Design review of the part built by this model. Coordinates are the model's own, in mm. Give positions to 0.01 mm unless a question says otherwise; leave off trailing zeros. Answer in a Markdown table with one row per item.
```python
from build123d import *

# Parameters (mm, degrees)
ESQUISSE1_W                                    = 381
ESQUISSE1_H                                    = 381
BOSS_EXTRU_1_DEPTH                             = 3
BOSS_EXTRU_2_DEPTH                             = 3
FRAISAGE_POUR_VIS_T_TE_FRAIS_E_M31_D           = 3.4
FRAISAGE_POUR_VIS_T_TE_FRAIS_E_M31_CSINK_D     = 6.3
FRAISAGE_POUR_VIS_T_TE_FRAIS_E_M31_CSINK_ANGLE = 90


with BuildPart() as part:
    # Esquisse1 → Boss.-Extru.1 (new body)
    with BuildSketch(Plane.XY):
        with Locations((190.5, 190.5)):
            Rectangle(ESQUISSE1_W, ESQUISSE1_H)
    extrude(amount=BOSS_EXTRU_1_DEPTH)

    # Esquisse2 → Boss.-Extru.2 (add)
    with BuildSketch(Plane.XY.offset(3)):
        with BuildLine():
            Line((6.5, 3.1), (374.5, 3.1))
            ThreePointArc((374.5, 3.1), (376.904163056, 4.095836944), (377.9, 6.5))
            Line((377.9, 6.5), (377.9, 374.5))
            ThreePointArc((377.9, 374.5), (376.904163056, 376.904163056), (374.5, 377.9))
            Line((374.5, 377.9), (6.5, 377.9))
            ThreePointArc((6.5, 377.9), (4.095836944, 376.904163056), (3.1, 374.5))
            Line((3.1, 374.5), (3.1, 6.5))
            ThreePointArc((3.1, 6.5), (4.095836944, 4.095836944), (6.5, 3.1))
        make_face()
    extrude(amount=BOSS_EXTRU_2_DEPTH)

    # Fraisage pour vis à tête fraisée M31 (through all)
    with Locations(Plane(origin=(0, 0, 0), x_dir=(-1, 0, 0), z_dir=(0, 0, -1))):
        with Locations((-28.5, 5), (-82.5, 5), (-136.5, 5), (-190.5, 5), (-244.5, 5), (-298.5, 5), (-352.5, 5), (-376, 28.5), (-376, 82.5), (-376, 136.5), (-376, 190.5), (-376, 244.5), (-376, 298.5), (-376, 352.5), (-352.5, 376), (-298.5, 376), (-244.5, 376), (-190.5, 376), (-136.5, 376), (-82.5, 376), (-28.5, 376), (-5, 352.5), (-5, 298.5), (-5, 244.5), (-5, 190.5), (-5, 136.5), (-5, 82.5), (-5, 28.5)):
            CounterSinkHole(FRAISAGE_POUR_VIS_T_TE_FRAIS_E_M31_D / 2, FRAISAGE_POUR_VIS_T_TE_FRAIS_E_M31_CSINK_D / 2, counter_sink_angle=FRAISAGE_POUR_VIS_T_TE_FRAIS_E_M31_CSINK_ANGLE)


solid = part.part
```
1) The part is to be moulded in two halves that separate along Z. For faces 1 (the face through (188, 193, 0)), 2 (the face through (188, 193, 6)), say which applies: released by +Z, released by -Z, zero draft, split by the parting line, or undercut.
Geometry says:
| item | result |
|---|---|
| face 1 | released by -Z |
| face 2 | released by +Z |
2) Insertion check: P1, Ø5.5, axis at x = 298.5, y = 376, coming from the +Z side; P2, Ø4.5, axis at x = 190.5, y = 376, coming from the -Z side; P3, Ø5.5, axis at x = 376, y = 82.5, coming from the -Z side. Each pin has a flat end and moves straight along its axis. Give the tip position at first contact, or say it passes through.
Geometry says:
| item | result |
|---|---|
| P1 | z = 6 |
| P2 | z = 0.9 |
| P3 | z = 0.4 |
3) To check wall thickness, follow probe 1 along Y at (x, z) = (190.5, 4.95); probe 2 along Y at (x, z) = (190.5, 2.75). State the ranges of each line that lie inside material, in increasing order. Write a range as [from, to].
Geometry says:
| item | result |
|---|---|
| probe 1 | [3.1, 3.3], [6.7, 374.3], [377.7, 377.9] |
| probe 2 | [0, 3.3], [6.7, 374.3], [377.7, 381] |
